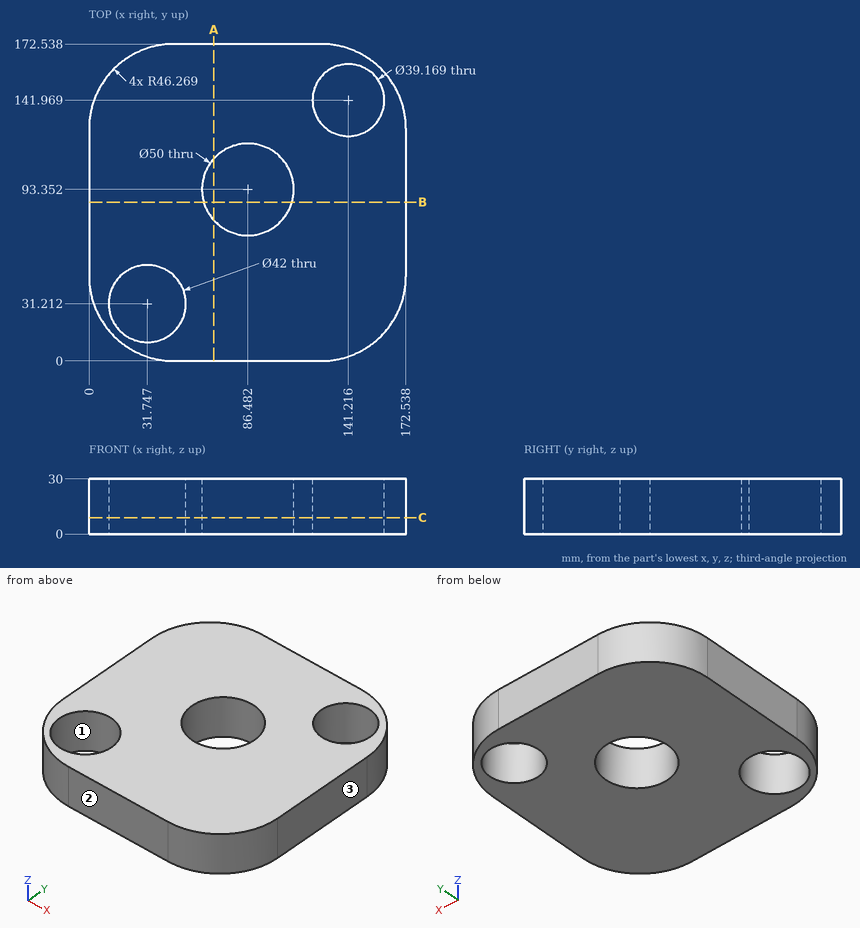
Can you work these out from the drawing? Everything is in mm from the part's minimum corner. Round coordinates to 2 decimals unless told otherwise and drop trailing zeros. Loops run counter-clockwise (first coordinate to the right, second up) from the corner with the lowest first, then second, coordinate; pieces in that order, holes last.
1. If we section it at A-A on x = 68: Write out the boundary of the cut face in (y, z).
Answer list:
outline: (0, 0) - (76.52, 0) - (76.52, 30) - (0, 30) - close; (110.19, 0) - (172.54, 0) - (172.54, 30) - (110.19, 30) - close
2. If we section it at C-C on z = 9: Write out the boundary of the cut face in (x, y) (1 decimal), plus the area to 3 significant figures.
Answer list:
outline: (0, 46.3) arc R46.3 ccw to (46.3, 0) - (126.3, 0) arc R46.3 ccw to (172.5, 46.3) - (172.5, 126.3) arc R46.3 ccw to (126.3, 172.5) - (46.3, 172.5) arc R46.3 ccw to (0, 126.3) - close; hole circle Ø42 at (31.7, 31.2); hole circle Ø50 at (86.5, 93.4); hole circle Ø39.2 at (141.2, 142)
area: 23,400 mm2
3. If I drill on line 1 along X through (y, z) = (48.5, 2) (1 decimal); line 2 along Y through (x, z) = (75.5, 3.5) (1 decimal); line 3 along X through (y, z) = (27.5, 21.5) (1 decimal), over which ranges is the centre line in solid material (lowest first)?
Answer list:
line 1: x = 0 to 19.8, 43.7 to 172.5
line 2: y = 0 to 70.9, 115.8 to 172.5
line 3: x = 4 to 11.1, 52.4 to 168.6
4. We'd pull the mould along Y, two halves only. Please class the marked faces 1, 2 and 3: +Y half, -Y half, draft (parallel to the pull), parting line (faces both ways), or undercut.
Answer list:
face 1: undercut
face 2: -Y half
face 3: draft
5. For P1, Ø2, axis at x = 152.5, z = 18.5, coming from the -Y side (1 decimal); P2, Ø8, axis at y = 146, z = 3.5, coming from the +X side; P3, Ø12, axis at x = 107.5, y = 110.5, coming from the -Z side, each with a flat end and sliding along its axis, tell me the tip position at first contact or that it passes through.
Answer list:
P1: stops at y = 7.5
P2: stops at x = 169.78
P3: stops at z = 0
6. If we section it at B-B on y = 86.5: Write out the boundary of the cut face in (x, z) (1 decimal).
Answer list:
outline: (0, 0) - (62.4, 0) - (62.4, 30) - (0, 30) - close; (110.5, 0) - (172.5, 0) - (172.5, 30) - (110.5, 30) - close
